CAD build for the part. Positions are in the model's coordinates, mm. A direction names the side the tool comes from. Round coordinates to 2 decimals unless told otherwise and drop trailing zeros. Loops run counter-clockwise (first coordinate to the right, second up) from the corner with the lowest first, then second, coordinate; pieces in that order, holes last.
```python
from build123d import *

# Parameters (mm, degrees)
SKETCH1_W               = 8
SKETCH1_H               = 8
BOSS_EXTRUDE1_DEPTH     = 3
CUT_EXTRUDE1_DEPTH      = 12.704699911
CUT_EXTRUDE1_DEPTH_BACK = 12.704699911
CUT_EXTRUDE2_DEPTH      = 11
SKETCH4_R               = 1.75
CUT_EXTRUDE3_DEPTH      = 0.4
SKETCH5_W               = 8
SKETCH5_H               = 1
BOSS_EXTRUDE2_DEPTH     = 2
FILLET1_R               = 4
CUT_EXTRUDE4_DEPTH      = 0.4
CUT_EXTRUDE5_DEPTH      = 0.5


with BuildPart() as part:
    # Sketch1 → Boss-Extrude1 (new body)
    with BuildSketch(Plane(origin=(0, 0, 0), x_dir=(1, 0, 0), z_dir=(0, 1, 0))):
        with Locations((4, 4)):
            Rectangle(SKETCH1_W, SKETCH1_H)
    extrude(amount=BOSS_EXTRUDE1_DEPTH)

    # Sketch2 → Cut-Extrude1 (cut, two sides: drawn at the far end of the back side and taken through both)
    with BuildSketch(Plane.XY.offset(-CUT_EXTRUDE1_DEPTH_BACK)):
        Polygon((0, 0), (0.6, 3), (0, 3), align=None)
        Polygon((8, 0), (7.4, 3), (8, 3), align=None)
    extrude(amount=CUT_EXTRUDE1_DEPTH + CUT_EXTRUDE1_DEPTH_BACK, mode=Mode.SUBTRACT)

    # Sketch3 → Cut-Extrude2 (cut)
    with BuildSketch(Plane(origin=(0, 0, 0), x_dir=(0, 0, -1), z_dir=(1, 0, 0))):
        Polygon((0, 0), (0.6, 3), (0, 3), align=None)
        Polygon((8, 3), (7.4, 3), (8, 0), align=None)
    extrude(amount=CUT_EXTRUDE2_DEPTH, mode=Mode.SUBTRACT)

    # Sketch4 → Cut-Extrude3 (cut)
    with BuildSketch(Plane.XZ):
        with Locations(Location((4, -3.75, 0), (0, 0, 270))):
            Circle(SKETCH4_R)
    extrude(amount=-CUT_EXTRUDE3_DEPTH, mode=Mode.SUBTRACT)

    # Sketch5 → Boss-Extrude2 (add)
    with BuildSketch(Plane.XZ):
        with Locations((4, -7.5)):
            Rectangle(SKETCH5_W, SKETCH5_H)
    extrude(amount=BOSS_EXTRUDE2_DEPTH)

    # Fillet1
    # the kernel refuses this fillet: 4 mm, written as the material it takes off along each edge
    with BuildSketch(Plane(origin=(8, -2, -16.660254038), x_dir=(0, 1, 0), z_dir=(0, 0, 1)), Plane(origin=(0, -2, 1.660254038), x_dir=(0, 1, 0), z_dir=(0, 0, -1))) as fillet1_piece_1:
        with BuildLine():
            CenterArc((4, 3.464101615), FILLET1_R, 180, 60)
            Line((0, 3.464101615), (-0.08, 3.464101615))
            Line((-0.08, 3.464101615), (-0.08, 0))
            Line((-0.08, 0), (0, -0.08))
            ThreePointArc((0, -0.08), (1, -0.08), (1.96, -0.069282032))
            Line((1.96, -0.069282032), (2, 0))
        make_face()
    extrude(amount=18.320508076, mode=Mode.SUBTRACT)

    # Sketch6 → Cut-Extrude4 (cut)
    with BuildSketch(Plane(origin=(0, 3, 0), x_dir=(1, 0, 0), z_dir=(0, 1, 0))):
        Polygon((2.459405501, 2.064543337), (2.459405501, 6.064543337), (3.22863627, 6.064543337), (3.22863627, 4.474799747), (4.869661911, 4.474799747), (4.869661911, 6.064543337), (5.63889268, 6.064543337), (5.63889268, 2.064543337), (4.869661911, 2.064543337), (4.869661911, 3.80813308), (3.22863627, 3.80813308), (3.22863627, 2.064543337), align=None)
    extrude(amount=-CUT_EXTRUDE4_DEPTH, mode=Mode.SUBTRACT)

    # Sketch7 → Cut-Extrude5 (cut)
    with BuildSketch(Plane(origin=(0, 3, 0), x_dir=(1, 0, 0), z_dir=(0, 1, 0))):
        Polygon((6.693034442, 1.488274187), (6.626528032, 1.86447611), (6.626528032, 2.206222905), (7.011143417, 2.206222905), (7.011143417, 1.86447611), (6.953451109, 1.488274187), align=None)
    extrude(amount=-CUT_EXTRUDE5_DEPTH, mode=Mode.SUBTRACT)


solid = part.part
```
Item 1: Cut at D-D, the plane x = 6. Give the cut face in (y, z).
Answers follow:
outline: (-1.72, -8) - (0, -8) - (3, -7.4) - (3, -0.6) - (0, 0) - (0, -7) - (-1.72, -7) - close
Item 2: Probe line 1 (X direction, y = 2.75, z = -3.5); line 2 (Y direction, x = 5.25, z = -1.5); line 3 (Z direction, x = 2.5, y = -1.2). List the from-to ranges inside material, lowest first.
Answers follow:
line 1: x = 0.55 to 2.46, 3.23 to 4.87, 5.64 to 7.45
line 2: y = 0 to 3
line 3: z = -8 to -7
Item 3: Flat gauge pins, fed straight in: P1, Ø1, axis at x = 6.5, z = -4.5, coming from the -Y side; P2, Ø1.5, axis at x = 6, y = 1.5, coming from the +Z side; P3, Ø0.6, axis at x = 2.5, y = -1, coming from the +Z side. Where does each tip first touch, or does it go through?
Answers follow:
P1: stops at y = 0
P2: stops at z = -0.15
P3: stops at z = -7
Item 4: Cut at B-B, the plane y = 0.7. Give the cut face in (x, z), plus the area to 3 significant figures.
Answers follow:
outline: (0.14, -7.86) - (7.86, -7.86) - (7.86, -0.14) - (0.14, -0.14) - close
area: 59.6 mm2
Item 5: Cut at A-A, the plane x = 4. Give the cut face in (y, z).
Answers follow:
outline: (-2, -8) - (0, -8) - (3, -7.4) - (3, -4.47) - (2.6, -4.47) - (2.6, -3.81) - (3, -3.81) - (3, -0.6) - (0, 0) - (0, -2) - (0.4, -2) - (0.4, -5.5) - (0, -5.5) - (0, -7) - (-2, -7) - close
Item 6: 3-axis set-ups, long thin cutter, end or side, ignore diameter. For faces 1 (the flat face through (4, 3, -5)), 2 (the cylindrical face through (2.94, 0.2, -2.36)), 3 (the flat face through (4, -1, -7)): which of +Z, -Z, +X, -X, +Y, -Y reach the whole face in a straight line?
Answers follow:
face 1: +Z, -Z, +X, -X, +Y
face 2: -Y
face 3: +Z, +X, -X, -Y
Item 7: Two-plate mould, pull along X, no slides. Class faces 4 (the flat face through (7.7, 1.5, -4.1)), 5 (the flat face through (0.3, 1.5, -4.1)), 6 (the flat face through (4, 2.6, -4)): released by +X, released by -X, zero draft, split by the parting line, or undercut.
Answers follow:
face 4: released by +X
face 5: released by -X
face 6: undercut
Item 8: Cut at C-C, the plane z = -1.25. Give the cut face in (x, y).
Answers follow:
outline: (0, 0) - (8, 0) - (7.4, 3) - (0.6, 3) - close
